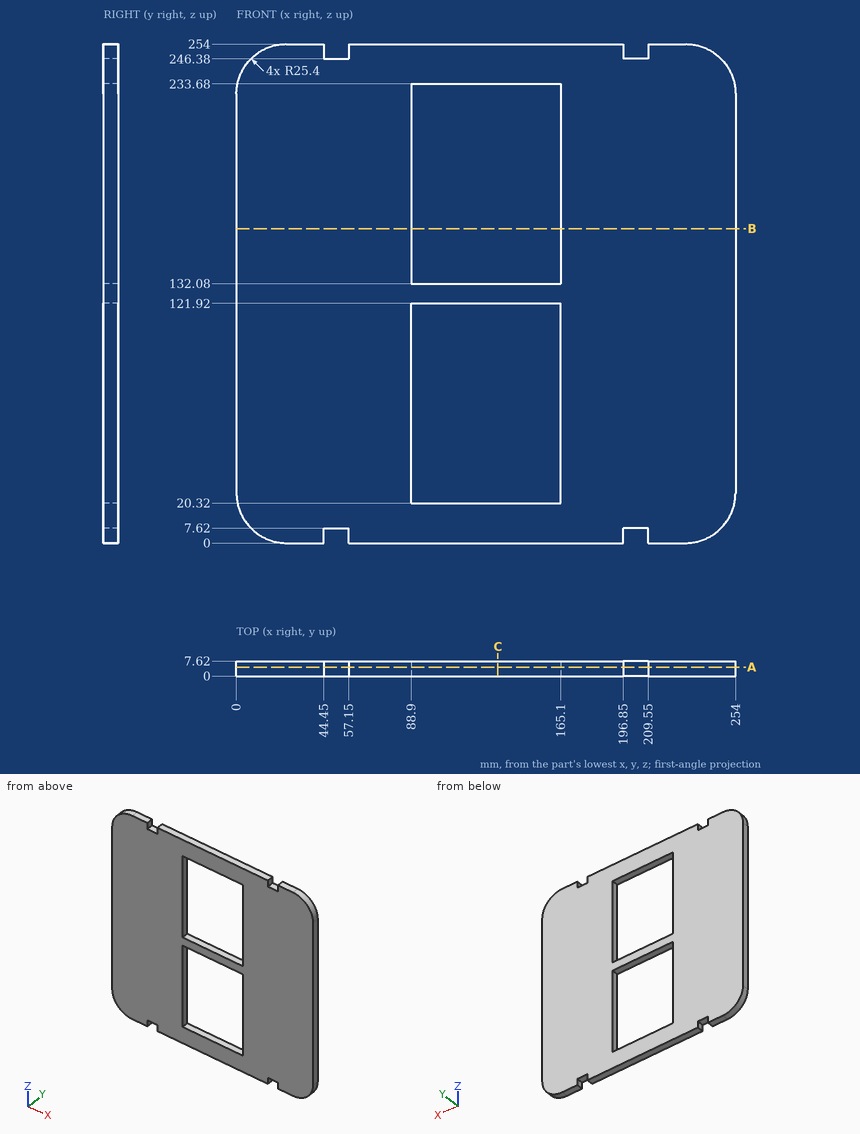
The figure shows three views and two pictorial views of one solid part (mm, origin at its lowest corner). Answer the questions. Give positions to 0.01 mm unless a question says otherwise; leave off trailing zeros. Write each loop counter-clockwise with the first axis right and the second up, starting at its lowest first coordinate (ties: lowest second). Pieces come first, ordered by that corner, then holes. Notation, with made-up numbers: (-11.5, 27.5) -> (15.5, 27.5) arc R20 cw to (15.5, 48.5) -> close; hole circle Ø8 at (24, 82). An arc over 180 degrees is marked (long way). Use one line per item in the form item = value.
1) Section B-B on z = 160 is taken. Write down the section's boundary in (x, y).
Result:
outline = (0, 0) -> (88.9, 0) -> (88.9, 7.62) -> (0, 7.62) -> close; (165.1, 0) -> (254, 0) -> (254, 7.62) -> (165.1, 7.62) -> close
2) Straight lines are drawn through the part: probe 1 along Z at (x, y) = (158.5, 3.5); probe 2 along X at (y, z) = (5.5, 156); probe 3 along Z at (x, y) = (230, 5.25). For each, find the intervals that lie inside material, in ascending order.
Result:
probe_1 = 0 to 20.32, 121.92 to 132.08, 233.68 to 254
probe_2 = 0 to 88.9, 165.1 to 254
probe_3 = 0.04 to 253.96
3) Section C-C on x = 133 is taken. Write down the section's boundary in (y, z), plus the area to 3 significant figures.
Result:
outline = (0, 0) -> (7.62, 0) -> (7.62, 20.32) -> (0, 20.32) -> close; (0, 121.92) -> (7.62, 121.92) -> (7.62, 132.08) -> (0, 132.08) -> close; (0, 233.68) -> (7.62, 233.68) -> (7.62, 254) -> (0, 254) -> close
area = 387 mm²
4) Section A-A on y = 4.5 is taken. Count the separate pieces of the cut face and the enclosed holes in it, plus the area to 3 significant figures.
Result:
separate_pieces = 1
enclosed_holes = 2
area = 48,100 mm²
5) Each of these flat-tipped pins is pushed along its axis until it touches: P1, Ø2, axis at x = 209.5, y = 6.5, coming from the -Z side; P2, Ø4, axis at y = 4.5, z = 4, coming from the +X side; P3, Ø2.5, axis at y = 3.5, z = 5, coming from the -X side; P4, Ø2.5, axis at x = 201, y = 2.5, coming from the -Z side. Where does it stop, or does it pass through?
Result:
P1 = 0
P2 = 245
P3 = 8.71
P4 = 7.62
